CAD build for the part. Positions are in the model's coordinates, mm. A direction names the side the tool comes from. Give positions to 0.01 mm unless a question says otherwise; leave off trailing zeros.
Item 1: Flat gauge pins, fed straight in: P1, Ø4, axis at y = 15, z = 113.5, coming from the +X side; P2, Ø4, axis at x = 7.5, y = -4, coming from the +Z side; P3, Ø2, axis at x = 0, z = 30, coming from the +Y side; P4, Ø8.5, axis at x = -16, z = 144.5, coming from the +Y side. Where does each tip first touch, or does it go through?
Item 2: Two-plate mould, pull along X, no slides. Class faces 1 (the cylindrical face through (-0.33, -20.988, 141.051)), 2 (the flat face through (-11.43, 0, 29)), 3 (the flat face through (5, -15, 133.325)): released by +X, released by -X, zero draft, split by the parting line, or undercut.
Item 3: Which spindle directions (+Z, -Z, +X, -X, +Y, -Y) get a long thin tool onto all of the face, cutting with end or side? Do faces 4 (the cylindrical face through (-0.33, -14.26, 3.76)), 5 (the flat face through (-16, -5.748, 145)), 6 (the flat face through (0, -18.999, 4)), 7 (the flat face through (-3.4, -11.2, 140.945)). Say none if no direction does.
Item 4: Band-saw the part on A-A on x = 0. Count the separate pieces of the cut face and the enclosed holes in it, plus the area to 3 significant figures.
Item 5: Wall check: L1, parallel to Y at x = 0, z = 139.95; L2, parallel to Z at x = 11.5, y = 17.5; L3, parallel to Z at x = -2.5, y = 9.5. Give the ranges that are in metal, low to high.
```python
from build123d import *

# Parameters (mm, degrees)
F2_W        = 22.86
F2_H        = 22.86
F2_R        = 11.24966
F11_DEPTH   = 2.54
F6_W        = 40.64
F6_H        = 24.13
F11_FACE_W  = 22.86
F11_FACE_H  = 22.86
F4_R        = 11.249914
F11_FACE1_W = 22.86
F11_FACE1_H = 22.86
F0_W        = 47.99838
F0_H        = 37.9984
F14_DEPTH   = 7.62
F16_R       = 14.986
F10_R       = 22.479
F10_R_2     = 14.986
F18_DEPTH   = 7.62
F19_DEPTH   = 7.62
F21_R       = 1.524
F22_DEPTH   = 25.4
F23_R       = 1.524
F24_DEPTH   = 25.4
F20_R       = 1.143
F25_DEPTH   = 25.4
F26_R       = 11.43
F27_DEPTH   = 1.99898


with BuildPart() as f11:
    # F2 (on offset) → F11 (new body)
    with BuildSketch(Plane.XY.offset(30.48)):
        Rectangle(F2_W, F2_H)
        Circle(F2_R, mode=Mode.SUBTRACT)
        Circle(F2_R)
    extrude(amount=-F11_DEPTH)

    # F6 (on offset) → F12 section 0
    with BuildSketch(Plane.XY.offset(7.62)):
        Rectangle(F6_W, F6_H)
    # F11_face (on face) → F12 section 1
    with BuildSketch(Plane(origin=(0, 0, 27.94), x_dir=(1, 0, 0), z_dir=(0, 0, -1))):
        Rectangle(F11_FACE_W, F11_FACE_H)
    loft()

    # F4 (on offset) → F13 section 0
    with BuildSketch(Plane.XY.offset(110.4646)):
        Circle(F4_R)
    # F11_face1 (on face) → F13 section 1
    with BuildSketch(Plane.XY.offset(30.48)):
        Rectangle(F11_FACE1_W, F11_FACE1_H)
    loft()

    # F0 (on Top) → F14 (join, through all)
    with BuildSketch(Plane.XY):
        Rectangle(F0_W, F0_H)
    extrude(amount=F14_DEPTH)

    # F13_face (on face) → F17 section 0
    with BuildSketch(Plane.XY.offset(110.4646)):
        with BuildLine():
            ThreePointArc((11.249914, 0), (10.3935652871, 4.3051557033), (7.9548904772, 7.9548904772))
            ThreePointArc((7.9548904772, 7.9548904772), (0, 11.249914), (-7.9548904772, 7.9548904772))
            ThreePointArc((-7.9548904772, 7.9548904772), (-11.249914, 0), (-7.9548904772, -7.9548904772))
            ThreePointArc((-7.9548904772, -7.9548904772), (0, -11.249914), (7.9548904772, -7.9548904772))
            ThreePointArc((7.9548904772, -7.9548904772), (10.3935652871, -4.3051557033), (11.249914, 0))
        make_face()
    # F16 (on offset) → F17 section 1
    with BuildSketch(Plane.XY.offset(133.3246)):
        Circle(F16_R)
    loft()

    # F10 (on offset) → F18 (join, through all)
    with BuildSketch(Plane.XY.offset(140.9446)):
        Circle(F10_R)
        Circle(F10_R_2, mode=Mode.SUBTRACT)
        Circle(F10_R_2)
    extrude(amount=-F18_DEPTH)

    # F8 (on offset) → F19 (join, through all)
    with BuildSketch(Plane.XY.offset(148.5646)):
        with BuildLine():
            ThreePointArc((-21.7316752019, -5.74802), (0, -22.479), (21.7316752019, -5.74802))
            Line((21.7316752019, -5.74802), (11.3247634006, -5.74802))
            ThreePointArc((11.3247634006, -5.74802), (0, -12.7), (-11.3247634006, -5.74802))
            Line((-11.3247634006, -5.74802), (-21.7316752019, -5.74802))
        make_face()
        with BuildLine():
            Line((11.3247634006, 5.74802), (21.7316752019, 5.74802))
            ThreePointArc((21.7316752019, 5.74802), (0, 22.479), (-21.7316752019, 5.74802))
            Line((-21.7316752019, 5.74802), (-11.3247634006, 5.74802))
            ThreePointArc((-11.3247634006, 5.74802), (0, 12.7), (11.3247634006, 5.74802))
        make_face()
    extrude(amount=-F19_DEPTH)

    # F21 (on face) → F22 (cut)
    with BuildSketch(Plane(origin=(0, 0, 0), x_dir=(1, 0, 0), z_dir=(0, 0, -1))):
        with Locations((-18.9992, 15.748)):
            Circle(F21_R)
        with Locations((0, 15.748)):
            Circle(F21_R)
        with Locations((18.9992, 15.748)):
            Circle(F21_R)
        with Locations((-18.9992, -15.748)):
            Circle(F21_R)
        with Locations((0, -15.748)):
            Circle(F21_R)
        with Locations((18.9992, -15.748)):
            Circle(F21_R)
    extrude(amount=-F22_DEPTH, mode=Mode.SUBTRACT)

    # F23 (on face) → F24 (cut)
    with BuildSketch(Plane.XY.offset(148.5646)):
        with Locations((0, 19.49958)):
            Circle(F23_R)
        with Locations((12.5543980573, 12.5543980573)):
            Circle(F23_R)
        with Locations((0, -19.499834)):
            Circle(F23_R)
        with Locations((-12.5543980573, -12.5543980573)):
            Circle(F23_R)
    extrude(amount=-F24_DEPTH, mode=Mode.SUBTRACT)

    # F20 (on face) → F25 (cut)
    with BuildSketch(Plane.XY.offset(140.9446)):
        with Locations((16.9926, 0)):
            Circle(F20_R)
        with Locations((-16.9926, 0)):
            Circle(F20_R)
    extrude(amount=-F25_DEPTH, mode=Mode.SUBTRACT)

    # F26 (on face) → F27 (cut)
    with BuildSketch(Plane.XY.offset(140.9446)):
        Circle(F26_R)
    extrude(amount=-F27_DEPTH, mode=Mode.SUBTRACT)


solid = f11.part
```
The answers:
1. P1: passes through
1. P2: stops at z = 138.95
1. P3: stops at y = 11.43
1. P4: stops at y = 19.16
2. face 1: undercut
2. face 2: released by -X
2. face 3: zero draft
3. face 4: -Z
3. face 5: +Z, +X, -X
3. face 6: -Z, +X, -X, -Y
3. face 7: +Z
4. separate pieces: 5
4. enclosed holes: 0
4. area: 3,550 mm2
5. L1: y = -22.48 to -21.02, -17.98 to -11.43, 11.43 to 17.98, 21.02 to 22.48
5. L2: z = 0 to 7.62, 133.32 to 148.56
5. L3: z = 0 to 138.95
